Here's how the part is built. I have some questions about the finished solid (model axes, mm). Coordinates: 2 decimals unless noted, no trailing zeros. Answer as a JSON object with one key per item and string values. Group by question number.
Q1. I want a section at A-A on y = -26.5. Count the separate pieces of the cut face and the enclosed holes in it, then the cut area to 3 significant figures.
Q2. I need wall thicknesses on line 1 (Y direction, x = -41.5, z = 11.75); line 2 (Y direction, x = -60, z = 8.5); line 3 (X direction, y = 55.5, z = 10.25). Which ranges of each line are inside material? Lowest first, please.
Q3. I'm going to push flat-ended pins straight in: pin 1 (0.5 mm diameter, centred on x = -41.5, y = 58, fed in from +Z); pin 2 (2 mm diameter, centred on x = -43, y = -29, fed in from -Z); pin 3 (1.5 mm diameter, centred on x = -56, y = -56, fed in from +Z). Where does each tip first touch, or does it pass through?
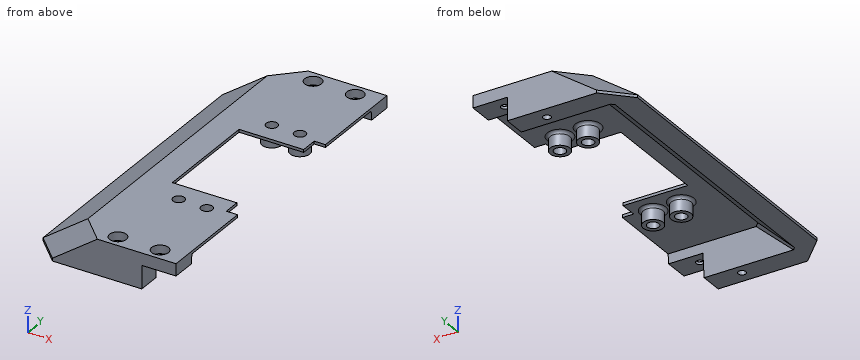
```python
from build123d import *
from build123d.topology import SkipClean

# Parameters (mm, degrees)
BOSS_EXTRUDE1_DEPTH = 1
SKETCH7_W           = 4
SKETCH7_H           = 50
CUT_EXTRUDE1_DEPTH  = 106.49052105
SKETCH8_W           = 12.2
SKETCH8_H           = 5.2
CUT_EXTRUDE2_DEPTH  = 149.162917235
SKETCH9_R           = 1.35
CUT_EXTRUDE3_DEPTH  = 106.604214081
SKETCH10_R          = 3
CUT_EXTRUDE4_DEPTH  = 3
CUT_EXTRUDE8_DEPTH  = 0.2
SKETCH15_W          = 2.7
SKETCH15_H          = 2.7
CUT_EXTRUDE9_DEPTH  = 0.2
SKETCH16_R          = 2.05
CUT_EXTRUDE10_DEPTH = 106.49052105
BOSS_EXTRUDE2_START = 5
SKETCH17_R          = 3.5
SKETCH17_R_2        = 2.05
BOSS_EXTRUDE2_DEPTH = 5
FILLET1_R           = 1
SKETCH18_W          = 5
SKETCH18_H          = 22
CUT_EXTRUDE11_DEPTH = 106.49052105
CUT_EXTRUDE12_REACH = 150.163
SKETCH19_W          = 12.2
SKETCH19_H          = 3
CUT_EXTRUDE13_REACH = 150.163
SKETCH20_W          = 12.2
SKETCH20_H          = 3
SKETCH23_R          = 1.35
CUT_EXTRUDE14_DEPTH = 106.604214081
SKETCH24_R          = 3
CUT_EXTRUDE15_DEPTH = 3
CUT_EXTRUDE16_DEPTH = 0.2
SKETCH26_W          = 2.7
SKETCH26_H          = 2.7
CUT_EXTRUDE17_DEPTH = 0.2
SKETCH27_W          = 23
SKETCH27_H          = 38
CUT_EXTRUDE18_DEPTH = 106.49052105


with BuildPart() as part:
    # Sketch2 → Boss-Extrude1 (new body)
    with BuildSketch(Plane.XY):
        Polygon((-86, -51), (-77, -60), (-33, -60), (-33, 60), (-77, 60), (-86, 51), align=None)
    extrude(amount=BOSS_EXTRUDE1_DEPTH)

    # Sketch4 → Loft1 section 0
    with BuildSketch(Plane.XY.offset(1)):
        with BuildLine():
            Line((-86, 51), (-86, -51))
            Line((-86, -51), (-77, -60))
            Line((-77, -60), (-33, -60))
            Line((-33, -60), (-33, 60))
            Line((-33, 60), (-77, 60))
            Line((-77, 60), (-86, 51))
        make_face()
    # Sketch3 → Loft1 section 1
    with BuildSketch(Plane.XY.offset(12.5)):
        with BuildLine():
            Line((-33, 60), (-61, 60))
            Line((-61, 60), (-70, 51))
            Line((-70, 51), (-70, -51))
            Line((-70, -51), (-61, -60))
            Line((-61, -60), (-33, -60))
            Line((-33, -60), (-33, 60))
        make_face()
    loft()

    # Sketch6 → Cut-Loft1 section 0
    with BuildSketch(Plane.XY.offset(11.5)):
        with BuildLine():
            Line((-33, 51), (-64.343145751, 51))
            Line((-64.343145751, 51), (-66, 49.343145751))
            Line((-66, 49.343145751), (-66, -49.343145751))
            Line((-66, -49.343145751), (-64.343145751, -51))
            Line((-64.343145751, -51), (-33, -51))
            Line((-33, -51), (-33, 51))
        make_face()
    # Sketch5 → Cut-Loft1 section 1
    with BuildSketch(Plane(origin=(0, 0, 0), x_dir=(-1, 0, 0), z_dir=(0, 0, -1))):
        with BuildLine():
            Line((33, 52), (77, 52))
            Line((77, 52), (78, 51))
            Line((78, 51), (78, -51))
            Line((78, -51), (77, -52))
            Line((77, -52), (33, -52))
            Line((33, -52), (33, 52))
        make_face()
    loft(mode=Mode.SUBTRACT)

    # Sketch7 → Cut-Extrude1 (cut, through all)
    with BuildSketch(Plane(origin=(0, 0, 11.5), x_dir=(-1, 0, 0), z_dir=(0, 0, -1))):
        with Locations((35, 0)):
            Rectangle(SKETCH7_W, SKETCH7_H)
    extrude(amount=-CUT_EXTRUDE1_DEPTH, mode=Mode.SUBTRACT)

    # Sketch8 → Cut-Extrude2 (cut, through all)
    with BuildSketch(Plane.XZ.offset(60)):
        with Locations((-39.1, 2.6)):
            Rectangle(SKETCH8_W, SKETCH8_H)
    extrude(amount=-CUT_EXTRUDE2_DEPTH, mode=Mode.SUBTRACT)

    # Sketch9 → Cut-Extrude3 (cut, through all)
    with BuildSketch(Plane.XY.offset(12.5)):
        with Locations((-41.5, 55.5)):
            Circle(SKETCH9_R)
        with Locations((-41.5, -55.5)):
            Circle(SKETCH9_R)
    extrude(amount=-CUT_EXTRUDE3_DEPTH, mode=Mode.SUBTRACT)

    # Sketch10 → Cut-Extrude4 (cut)
    with BuildSketch(Plane.XY.offset(12.5)):
        with Locations((-41.5, 55.5)):
            Circle(SKETCH10_R)
        with Locations((-41.5, -55.5)):
            Circle(SKETCH10_R)
    extrude(amount=-CUT_EXTRUDE4_DEPTH, mode=Mode.SUBTRACT)

    # Sketch14 → Cut-Extrude8 (cut)
    with SkipClean():  # the faces are left unmerged after this step: merging them gives an invalid solid
        with BuildSketch(Plane.XY.offset(9.5)):
            with BuildLine():
                Line((-42.85, -58.179085665), (-42.85, -52.820914335))
                ThreePointArc((-42.85, -52.820914335), (-41.5, -52.5), (-40.15, -52.820914335))
                Line((-40.15, -52.820914335), (-40.15, -58.179085665))
                ThreePointArc((-40.15, -58.179085665), (-41.5, -58.5), (-42.85, -58.179085665))
            make_face()
        cut_extrude8 = extrude(amount=-CUT_EXTRUDE8_DEPTH, mode=Mode.SUBTRACT)

    # Sketch15 → Cut-Extrude9 (cut)
    with SkipClean():  # the faces are left unmerged after this step: merging them gives an invalid solid
        with BuildSketch(Plane.XY.offset(9.3)):
            with Locations((-41.5, -55.5)):
                Rectangle(SKETCH15_W, SKETCH15_H)
        cut_extrude9 = extrude(amount=-CUT_EXTRUDE9_DEPTH, mode=Mode.SUBTRACT)

    # Mirror1: Cut-Extrude8, Cut-Extrude9 across plane
    with SkipClean():  # the faces are left unmerged after this step: merging them gives an invalid solid
        add(cut_extrude8.mirror(Plane.ZX), mode=Mode.SUBTRACT)
        add(cut_extrude9.mirror(Plane.ZX), mode=Mode.SUBTRACT)

    # Sketch16 → Cut-Extrude10 (cut, through all)
    with SkipClean():  # the faces are left unmerged after this step: merging them gives an invalid solid
        with BuildSketch(Plane(origin=(0, 0, 11.5), x_dir=(-1, 0, 0), z_dir=(0, 0, -1))):
            with Locations((43, 26.5)):
                Circle(SKETCH16_R)
            with Locations((53, 26.5)):
                Circle(SKETCH16_R)
            with Locations((53, -26.5)):
                Circle(SKETCH16_R)
            with Locations((43, -26.5)):
                Circle(SKETCH16_R)
        extrude(amount=-CUT_EXTRUDE10_DEPTH, mode=Mode.SUBTRACT)

    # Sketch17 → Boss-Extrude2 (add)
    # profile 1 of 4: a face of its own
    with SkipClean():  # the faces are left unmerged after this step: merging them gives an invalid solid
        with BuildSketch(Plane(origin=(0, 0, 11.5), x_dir=(-1, 0, 0), z_dir=(0, 0, -1)).offset(BOSS_EXTRUDE2_START)):
            with Locations(Location((43, 26.5, 0), (0, 0, 180))):
                Circle(SKETCH17_R)
            with Locations((43, 26.5)):
                Circle(SKETCH17_R_2, mode=Mode.SUBTRACT)
        # profile 2 of 4: a face of its own
        with BuildSketch(Plane(origin=(0, 0, 11.5), x_dir=(-1, 0, 0), z_dir=(0, 0, -1)).offset(BOSS_EXTRUDE2_START)):
            with Locations(Location((53, 26.5, 0), (0, 0, 180))):
                Circle(SKETCH17_R)
            with Locations((53, 26.5)):
                Circle(SKETCH17_R_2, mode=Mode.SUBTRACT)
        # profile 3 of 4: a face of its own
        with BuildSketch(Plane(origin=(0, 0, 11.5), x_dir=(-1, 0, 0), z_dir=(0, 0, -1)).offset(BOSS_EXTRUDE2_START)):
            with Locations(Location((53, -26.5, 0), (0, 0, 180))):
                Circle(SKETCH17_R)
            with Locations((53, -26.5)):
                Circle(SKETCH17_R_2, mode=Mode.SUBTRACT)
        # profile 4 of 4: a face of its own
        with BuildSketch(Plane(origin=(0, 0, 11.5), x_dir=(-1, 0, 0), z_dir=(0, 0, -1)).offset(BOSS_EXTRUDE2_START)):
            with Locations(Location((43, -26.5, 0), (0, 0, 180))):
                Circle(SKETCH17_R)
            with Locations((43, -26.5)):
                Circle(SKETCH17_R_2, mode=Mode.SUBTRACT)
        extrude(amount=-BOSS_EXTRUDE2_DEPTH)

    # Fillet1
    fillet1_edges = [part.edges().sort_by_distance(p)[0] for p in [
        (-46.5, 26.5, 11.5),
        (-56.5, 26.5, 11.5),
        (-56.5, -26.5, 11.5),
        (-46.5, -26.5, 11.5),
    ]]
    fillet(fillet1_edges, radius=FILLET1_R)

    # Sketch18 → Cut-Extrude11 (cut, through all)
    with SkipClean():  # the faces are left unmerged after this step: merging them gives an invalid solid
        with BuildSketch(Plane(origin=(0, 0, 11.5), x_dir=(-1, 0, 0), z_dir=(0, 0, -1))):
            with Locations((39.5, 0)):
                Rectangle(SKETCH18_W, SKETCH18_H)
        extrude(amount=-CUT_EXTRUDE11_DEPTH, mode=Mode.SUBTRACT)

    # Cut-Extrude12: up to this plane
    with SkipClean():  # the faces are left unmerged after this step: merging them gives an invalid solid
        cut_extrude12_end = Plane(origin=(0, 51.609756098, 4.487804878), z_dir=(0, -0.9962405881956831, -0.08662961636484208))
        # Sketch19 → Cut-Extrude12 (cut, up to the surface)
        with BuildSketch(Plane(origin=(0, 60, 0), x_dir=(1, 0, 0), z_dir=(0, 1, 0)), mode=Mode.PRIVATE) as cut_extrude12_sk1:
            with Locations((-39.1, -6.7)):
                Rectangle(SKETCH19_W, SKETCH19_H)
        cut_extrude12_tool1 = split(extrude(cut_extrude12_sk1.sketch, amount=-CUT_EXTRUDE12_REACH, mode=Mode.PRIVATE), bisect_by=cut_extrude12_end, keep=Keep.BOTH, mode=Mode.PRIVATE)
        add(cut_extrude12_tool1.solids().sort_by_distance((-39.1, 60, 6.7))[0], mode=Mode.SUBTRACT)

    # Cut-Extrude13: up to this plane
    with SkipClean():  # the faces are left unmerged after this step: merging them gives an invalid solid
        cut_extrude13_end = Plane(origin=(0, -51.609756098, 4.487804878), z_dir=(0, -0.9962405881956831, 0.0866296163648415))
        # Sketch20 → Cut-Extrude13 (cut, up to the surface)
        with BuildSketch(Plane.XZ.offset(60), mode=Mode.PRIVATE) as cut_extrude13_sk1:
            with Locations((-39.1, 6.7)):
                Rectangle(SKETCH20_W, SKETCH20_H)
        cut_extrude13_tool1 = split(extrude(cut_extrude13_sk1.sketch, amount=-CUT_EXTRUDE13_REACH, mode=Mode.PRIVATE), bisect_by=cut_extrude13_end, keep=Keep.BOTH, mode=Mode.PRIVATE)
        add(cut_extrude13_tool1.solids().sort_by_distance((-39.1, -60, 6.7))[0], mode=Mode.SUBTRACT)

    # Sketch23 → Cut-Extrude14 (cut, symmetric)
    with SkipClean():  # the faces are left unmerged after this step: merging them gives an invalid solid
        with BuildSketch(Plane.XY.offset(12.5)):
            with Locations((-56.5, -55.5)):
                Circle(SKETCH23_R)
        cut_extrude14 = extrude(amount=CUT_EXTRUDE14_DEPTH, both=True, mode=Mode.SUBTRACT)

    # Sketch24 → Cut-Extrude15 (cut)
    with SkipClean():  # the faces are left unmerged after this step: merging them gives an invalid solid
        with BuildSketch(Plane.XY.offset(12.5)):
            with Locations((-56.5, -55.5)):
                Circle(SKETCH24_R)
        cut_extrude15 = extrude(amount=-CUT_EXTRUDE15_DEPTH, mode=Mode.SUBTRACT)

    # Sketch25 → Cut-Extrude16 (cut)
    with SkipClean():  # the faces are left unmerged after this step: merging them gives an invalid solid
        with BuildSketch(Plane.XY.offset(9.5)):
            with BuildLine():
                Line((-57.85, -58.179085665), (-57.85, -52.820914335))
                ThreePointArc((-57.85, -52.820914335), (-56.5, -52.5), (-55.15, -52.820914335))
                Line((-55.15, -52.820914335), (-55.15, -58.179085665))
                ThreePointArc((-55.15, -58.179085665), (-56.5, -58.5), (-57.85, -58.179085665))
            make_face()
        cut_extrude16 = extrude(amount=-CUT_EXTRUDE16_DEPTH, mode=Mode.SUBTRACT)

    # Sketch26 → Cut-Extrude17 (cut)
    with SkipClean():  # the faces are left unmerged after this step: merging them gives an invalid solid
        with BuildSketch(Plane.XY.offset(9.3)):
            with Locations((-56.5, -55.5)):
                Rectangle(SKETCH26_W, SKETCH26_H)
        cut_extrude17 = extrude(amount=-CUT_EXTRUDE17_DEPTH, mode=Mode.SUBTRACT)

    # Mirror2: Cut-Extrude14, Cut-Extrude15, Cut-Extrude16, Cut-Extrude17 across plane
    with SkipClean():  # the faces are left unmerged after this step: merging them gives an invalid solid
        add(cut_extrude14.mirror(Plane.ZX), mode=Mode.SUBTRACT)
        add(cut_extrude15.mirror(Plane.ZX), mode=Mode.SUBTRACT)
        add(cut_extrude16.mirror(Plane.ZX), mode=Mode.SUBTRACT)
        add(cut_extrude17.mirror(Plane.ZX), mode=Mode.SUBTRACT)

    # Sketch27 → Cut-Extrude18 (cut, through all)
    with SkipClean():  # the faces are left unmerged after this step: merging them gives an invalid solid
        with BuildSketch(Plane(origin=(0, 0, 11.5), x_dir=(-1, 0, 0), z_dir=(0, 0, -1))):
            with Locations((48.5, 0)):
                Rectangle(SKETCH27_W, SKETCH27_H)
        extrude(amount=-CUT_EXTRUDE18_DEPTH, mode=Mode.SUBTRACT)


solid = part.part
```
Result set:
{
 "1": {"separate pieces": "3", "enclosed holes": "0", "area": "144 mm²"},
 "2": {"line 1": "y = -60 to -58.5, -52.5 to -27.9, -25.1 to -19, 19 to 25.1, 27.9 to 52.5, 58.5 to 60", "line 2": "y = -60 to -51.26, 51.26 to 60", "line 3": "x = -68.63 to -59.5, -53.5 to -44.5, -38.5 to -33"},
 "3": {"pin 1": "stops at z = 9.3", "pin 2": "stops at z = 6.5", "pin 3": "stops at z = 9.1"}
}
